Input: part model. Units: mm. Frame: model coordinates. A direction names the side the tool comes from. Coordinates: 2 decimals unless noted, no trailing zeros. Order: outer loops, then holes, each group sorted by start corner. A loop starts at its lowest first (then second) coordinate and runs counter-clockwise, first axis right, second up. Notation, with made-up numbers: (67.25, 21) - (86.25, 21) arc R25 ccw to (86.25, 59) - close; hole circle Ø4 at (8, 14). An arc over 180 degrees is marked (long way). Answer as CSV lines item,"result". Start each with the question number.
Item 1: Section B-B (x = 0). Output: boundary loops of the cut face in (y, z) (3 decimals), and give its area (3 significant figures).
Item 2: Section C-C (y = 1.75). Output: boundary loops of the cut face in (x, z) (3 decimals), and give its area (3 significant figures).
Item 3: Access query for faces 4 (the cylindrical face through (18.705, 1.878, 1.487)), 5 (the conical face through (28.54, 9.55, -26.79)). Directions: +Z, -Z, +X, -X, +Y, -Y. A direction counts if a zero-diameter tool reaches every point of the face in a straight line with its end or side. Return the directions, or none.
Item 4: Draft query along Z for faces 1 (the cylindrical face through (-25.989, 6.439, -23.084)), 2 (the flat face through (38.1, 6, 0)), 3 (the cylindrical face through (37.336, 6.439, -37.376)). Return one class per face: +Z half, -Z half, draft (parallel to the pull), parting line (faces both ways), or undercut.
Item 5: Section A-A (z = 0). Output: boundary loops of the cut face in (x, y) (3 decimals).
Item 6: Material intervals for line 1 along X through (y, z) = (9, 0) (3 decimals); line 2 along X through (y, z) = (0.5, -27); line 3 along Z through (x, y) = (24, 5), sorted ascending.
Item 7: Section D-D (y = 11). Output: boundary loops of the cut face in (x, z) (3 decimals).
Item 8: First-contact query: pin 1 (1.4 mm diameter, centred on x = 27.5, z = -28, fed in from +Y). Flat tip, straight axial feed; report the tip coordinate or a pass-through.
from build123d import *

# Parameters (mm, degrees)
SKETCH1_W           = 76.2
SKETCH1_H           = 76.2
BOSS_EXTRUDE1_DEPTH = 12.7
CUT_EXTRUDE1_REACH  = 57.358
SKETCH2_R           = 4.445
CUT_EXTRUDE2_REACH  = 57.358
SKETCH6_R           = 4.445
SKETCH7_R           = 4.445
CUT_EXTRUDE3_DEPTH  = 3.81
CUT_EXTRUDE3_DRAFT  = -45
CUT_EXTRUDE4_REACH  = 57.358
SKETCH12_R          = 4.445
SKETCH13_R          = 6.858
CUT_EXTRUDE5_DEPTH  = 3.81
FILLET1_R           = 2.54


with BuildPart() as part:
    # Sketch1 → Boss-Extrude1 (new body)
    with BuildSketch(Plane(origin=(0, 0, 0), x_dir=(1, 0, 0), z_dir=(0, 1, 0))):
        Rectangle(SKETCH1_W, SKETCH1_H)
    extrude(amount=BOSS_EXTRUDE1_DEPTH)

    # Sketch2 → Cut-Extrude1 (cut, up to next)
    with BuildSketch(Plane.XZ, mode=Mode.PRIVATE) as cut_extrude1_sk1:
        with Locations(Location((0, 0, 0), (0, 0, 270))):
            Circle(SKETCH2_R)
    cut_extrude1_tool1 = extrude(cut_extrude1_sk1.sketch, amount=-CUT_EXTRUDE1_REACH, mode=Mode.PRIVATE) & part.part
    add(cut_extrude1_tool1.solids().sort_by_distance((0, 0, 0))[0], mode=Mode.SUBTRACT)

    # Sketch6 → Cut-Extrude2 (cut, up to next)
    with BuildSketch(Plane(origin=(0, 12.7, 0), x_dir=(1, 0, 0), z_dir=(0, 1, 0)), mode=Mode.PRIVATE) as cut_extrude2_sk1:
        with Locations(Location((-27.323692655, 27.323692655, 0), (0, 0, 270))):
            Circle(SKETCH6_R)
    cut_extrude2_tool1 = extrude(cut_extrude2_sk1.sketch, amount=-CUT_EXTRUDE2_REACH, mode=Mode.PRIVATE) & part.part
    # Sketch6 → Cut-Extrude2 (cut, up to next)
    with BuildSketch(Plane(origin=(0, 12.7, 0), x_dir=(1, 0, 0), z_dir=(0, 1, 0)), mode=Mode.PRIVATE) as cut_extrude2_sk2:
        with Locations(Location((27.323692655, -27.323692655, 0), (0, 0, 270))):
            Circle(SKETCH6_R)
    cut_extrude2_tool2 = extrude(cut_extrude2_sk2.sketch, amount=-CUT_EXTRUDE2_REACH, mode=Mode.PRIVATE) & part.part
    add(cut_extrude2_tool1.solids().sort_by_distance((-27.323693, 12.7, -27.323693))[0], mode=Mode.SUBTRACT)
    add(cut_extrude2_tool2.solids().sort_by_distance((27.323693, 12.7, 27.323693))[0], mode=Mode.SUBTRACT)


with BuildPart() as cut_extrude3_tool:
    # Sketch7 → Cut-Extrude3 (with draft: the straight prism first)
    with BuildSketch(Plane(origin=(0, 12.7, 0), x_dir=(1, 0, 0), z_dir=(0, 1, 0))):
        with Locations((27.94, 27.94)):
            Circle(SKETCH7_R)
    extrude(amount=-CUT_EXTRUDE3_DEPTH)
    # Cut-Extrude3: the draft: its side faces are tilted about the plane it starts from
    cut_extrude3_sides = [cut_extrude3_tool.faces().sort_by_distance(p)[0] for p in [
        (23.495, 10.795, -27.94),
    ]]
    draft(cut_extrude3_sides, Plane(origin=(0, 12.7, 0), x_dir=(1, 0, 0), z_dir=(0, 1, 0)), CUT_EXTRUDE3_DRAFT)


with BuildPart() as part_1:
    add(part.part)

    # Cut-Extrude3: cut by cut_extrude3_tool
    add(cut_extrude3_tool.part, mode=Mode.SUBTRACT)

    # Sketch12 → Cut-Extrude4 (cut, up to next)
    with BuildSketch(Plane(origin=(0, 12.7, 0), x_dir=(1, 0, 0), z_dir=(0, 1, 0)), mode=Mode.PRIVATE) as cut_extrude4_sk1:
        with Locations(Location((0, 25.4, 0), (0, 0, 270))):
            Circle(SKETCH12_R)
    cut_extrude4_tool1 = extrude(cut_extrude4_sk1.sketch, amount=-CUT_EXTRUDE4_REACH, mode=Mode.PRIVATE) & part_1.part
    # Sketch12 → Cut-Extrude4 (cut, up to next)
    with BuildSketch(Plane(origin=(0, 12.7, 0), x_dir=(1, 0, 0), z_dir=(0, 1, 0)), mode=Mode.PRIVATE) as cut_extrude4_sk2:
        with Locations(Location((25.4, 0, 0), (0, 0, 270))):
            Circle(SKETCH12_R)
    cut_extrude4_tool2 = extrude(cut_extrude4_sk2.sketch, amount=-CUT_EXTRUDE4_REACH, mode=Mode.PRIVATE) & part_1.part
    add(cut_extrude4_tool1.solids().sort_by_distance((0, 12.7, -25.4))[0], mode=Mode.SUBTRACT)
    add(cut_extrude4_tool2.solids().sort_by_distance((25.4, 12.7, 0))[0], mode=Mode.SUBTRACT)

    # Sketch13 → Cut-Extrude5 (cut)
    with BuildSketch(Plane.XZ):
        with Locations(Location((0, -25.4, 0), (0, 0, 270))):
            Circle(SKETCH13_R)
        with Locations(Location((25.4, 0, 0), (0, 0, 270))):
            Circle(SKETCH13_R)
    extrude(amount=-CUT_EXTRUDE5_DEPTH, mode=Mode.SUBTRACT)

    # Fillet1
    fillet1_edges = [part_1.edges().sort_by_distance(p)[0] for p in [
        (38.1, 6.35, 38.1),
        (-38.1, 6.35, 38.1),
        (-38.1, 6.35, -38.1),
        (38.1, 6.35, -38.1),
    ]]
    fillet(fillet1_edges, radius=FILLET1_R)


solid = part_1.part
Determined:
1,outline,"(0, -38.1) - (12.7, -38.1) - (12.7, -29.845) - (3.81, -29.845) - (3.81, -32.258) - (0, -32.258) - close; (0, -18.542) - (3.81, -18.542) - (3.81, -20.955) - (12.7, -20.955) - (12.7, -4.445) - (0, -4.445) - close; (0, 4.445) - (12.7, 4.445) - (12.7, 38.1) - (0, 38.1) - close"
1,area,"724 mm^2"
2,outline,"(-38.1, -35.56) arc R2.54 ccw to (-35.56, -38.1) - (35.56, -38.1) arc R2.54 ccw to (38.1, -35.56) - (38.1, 35.56) arc R2.54 ccw to (35.56, 38.1) - (-35.56, 38.1) arc R2.54 ccw to (-38.1, 35.56) - close; hole circle Ø8.89 at (-27.324, -27.324); hole circle Ø13.716 at (0, -25.4); hole circle Ø8.89 at (0, 0); hole circle Ø13.716 at (25.4, 0); hole circle Ø8.89 at (27.324, 27.324)"
2,area,"5,320 mm^2"
3,face 4,"-Y"
3,face 5,"+Y"
4,face 1,"undercut"
4,face 2,"draft"
4,face 3,"-Z half"
5,outline,"(-38.1, 0) - (-4.445, 0) - (-4.445, 12.7) - (-38.1, 12.7) - close; (4.445, 0) - (18.542, 0) - (18.542, 3.81) - (20.955, 3.81) - (20.955, 12.7) - (4.445, 12.7) - close; (29.845, 3.81) - (32.258, 3.81) - (32.258, 0) - (38.1, 0) - (38.1, 12.7) - (29.845, 12.7) - close"
6,line 1,"x = -38.1 to -4.445, 4.445 to 20.955, 29.845 to 38.1"
6,line 2,"x = -38.1 to -31.76, -22.89 to -6.67, 6.67 to 38.1"
6,line 3,"z = -38.1 to -4.22, 4.22 to 24.37, 30.28 to 38.1"
7,outline,"(-38.1, -35.56) arc R2.54 ccw to (-35.56, -38.1) - (35.56, -38.1) arc R2.54 ccw to (38.1, -35.56) - (38.1, 35.56) arc R2.54 ccw to (35.56, 38.1) - (-35.56, 38.1) arc R2.54 ccw to (-38.1, 35.56) - close; hole circle Ø8.89 at (-27.324, -27.324); hole circle Ø8.89 at (0, -25.4); hole circle Ø8.89 at (0, 0); hole circle Ø8.89 at (25.4, 0); hole circle Ø8.89 at (27.324, 27.324); hole circle Ø5.49 at (27.94, -27.94)"
8,pin 1,"stops at y = 9.4"
